```python
from build123d import *

# Parameters (mm, degrees)
BOSS_EXTRUDE1_DEPTH = 47
SKETCH3_R           = 4.75
SKETCH3_W           = 43.5
SKETCH3_H           = 6.5
CUT_EXTRUDE1_DEPTH  = 10


with BuildPart() as part:
    # Sketch2 → Boss-Extrude1 (new body)
    with BuildSketch(Plane(origin=(0, 0, 0), x_dir=(1, 0, 0), z_dir=(0, 1, 0))):
        Polygon((-43, 58), (43, 58), (58, 43), (58, -43), (43, -58), (-43, -58), (-58, -43), (-58, 43), align=None)
    extrude(amount=BOSS_EXTRUDE1_DEPTH)

    # Sketch3 → Cut-Extrude1 (cut)
    with BuildSketch(Plane.XY.offset(58)):
        with Locations((-23.75, 22.55)):
            Circle(SKETCH3_R)
        with Locations((0, 9.35)):
            Rectangle(SKETCH3_W, SKETCH3_H)
    extrude(amount=-CUT_EXTRUDE1_DEPTH, mode=Mode.SUBTRACT)


solid = part.part
```
Design review of the part built by this model. Coordinates are the model's own, in mm. A direction names the side the tool comes from. Round coordinates to 2 decimals unless told otherwise and drop trailing zeros. Write each loop counter-clockwise with the first axis right and the second up, starting at its lowest first coordinate (ties: lowest second). Pieces come first, ordered by that corner, then holes. Notation, with made-up numbers: (48, 57.25) -> (61, 57.25) arc R19 ccw to (61, 82.25) -> close; hole circle Ø4 at (17, -22). An arc over 180 degrees is marked (long way). Write item = value, one per line. Start each with the question number.
1) Mouldability with a two-part tool opening along Y and no side actions: class faces 1 (the face through (-1, 23, -58)), 2 (the face through (0, 9, 48)), 3 (the face through (21.75, 9, 53)), 4 (the face through (1, 0, -1)) as +Y half, -Y half, draft (parallel to the pull), parting line (faces both ways), or undercut.
2) Wall thickness on probe 1 along Y at (x, z) = (-23.75, 55.5); probe 2 along Y at (x, z) = (-23, 54); probe 3 along X at (y, z) = (22, 53): over which ranges is each line inside the solid? List them lowest first. Write a range as from..to.
3) Tool access review of faces 5 (the face through (-24, 23, 48)), 6 (the face through (58, 23, -1)): name each direction out of +Z, -Z, +X, -X, +Y, -Y from which nothing blocks a thin tool from reaching the whole face with its end or side.
4) Clearance check with flat-ended pins moving along their axes: pin 1 (7 mm diameter, centred on y = 9.5, z = 53.5, fed in from +X); pin 2 (7 mm diameter, centred on y = 9, z = 54.5, fed in from -X); pin 3 (2 mm diameter, centred on x = 5, y = 10.5, fed in from +Z). State where each tip first meets the part, or that it passes through.
5) Take a section at B-B, the plane x = -23.75. State the section outline as (y, z) points.
6) Take a section at A-A, the plane y = 39.5. State the section outline as (x, z) points, plus the area to 3 significant figures.
7) Take a section at D-D, the plane y = 22.55. State the section outline as (x, z) points.
8) Take a section at C-C, the plane y = 8.5. State the section outline as (x, z) points.
Results list:
q1.face_1 = draft
q1.face_2 = undercut
q1.face_3 = undercut
q1.face_4 = -Y half
q2.probe_1 = 0..17.8, 27.3..47
q2.probe_2 = 0..17.86, 27.24..47
q2.probe_3 = -48..-28.47, -19.03..48
q3.face_5 = +Z
q3.face_6 = +Z, -Z, +X, +Y, -Y
q4.pin_1 = 51
q4.pin_2 = -50
q4.pin_3 = 48
q5.outline = (0, -58) -> (47, -58) -> (47, 58) -> (27.3, 58) -> (27.3, 48) -> (17.8, 48) -> (17.8, 58) -> (0, 58) -> close
q6.outline = (-58, -43) -> (-43, -58) -> (43, -58) -> (58, -43) -> (58, 43) -> (43, 58) -> (-43, 58) -> (-58, 43) -> close
q6.area = 13,000 mm²
q7.outline = (-58, -43) -> (-43, -58) -> (43, -58) -> (58, -43) -> (58, 43) -> (43, 58) -> (-19, 58) -> (-19, 48) -> (-28.5, 48) -> (-28.5, 58) -> (-43, 58) -> (-58, 43) -> close
q8.outline = (-58, -43) -> (-43, -58) -> (43, -58) -> (58, -43) -> (58, 43) -> (43, 58) -> (21.75, 58) -> (21.75, 48) -> (-21.75, 48) -> (-21.75, 58) -> (-43, 58) -> (-58, 43) -> close
